from build123d import *

# Parameters (mm, degrees)
EXTRUDE_1_DEPTH     = 20
SKETCH_2_R          = 5
CUT_EXTRUDE_1_DEPTH = 18
CHAMFER_1_SIZE      = 3


with BuildPart() as part:
    # 草圖1 → 填料-伸長1 (new body)
    with BuildSketch(Plane(origin=(0, 0, 0), x_dir=(1, 0, 0), z_dir=(0, 1, 0))):
        Polygon((0, 0), (0, -20), (3.257359313, -23.257359313), (7.5, -19.014718626), (11.742640687, -23.257359313), (15, -20), (15, 0), align=None)
    extrude(amount=EXTRUDE_1_DEPTH)

    # 草圖2 → 除料-伸長1 (cut)
    with BuildSketch(Plane(origin=(0, 0, 0), x_dir=(-1, 0, 0), z_dir=(0, 0, -1))):
        with Locations((-7.5, 10)):
            Circle(SKETCH_2_R)
    extrude(amount=-CUT_EXTRUDE_1_DEPTH, mode=Mode.SUBTRACT)

    # 導角1
    chamfer_1_edges = [part.edges().sort_by_distance(p)[0] for p in [
        (7.5, 20, 0),
        (7.5, 0, 0),
    ]]
    chamfer(chamfer_1_edges, length=CHAMFER_1_SIZE)


solid = part.part
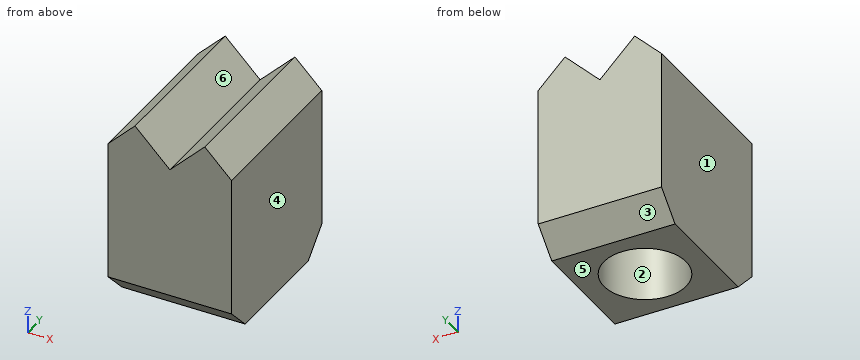
The model under review builds one solid part; all positions refer to its coordinate system, in mm. Face numbers are marked on the shaded views. A direction names the side the tool comes from. Round coordinates to 2 decimals unless told otherwise and drop trailing zeros. Loops run counter-clockwise (first coordinate to the right, second up) from the corner with the lowest first, then second, coordinate; pieces in that order, holes last. Notation, with made-up numbers: M 48.25,24.25 L 87.25,24.25 A26 ccw 87.25,41.25 Z; hole C 82,-16.5 d7. An arc over 180 degrees is marked long. Answer as CSV lines item,"result".
1. For the marked faces 5 and 6, list the 3-axis set-ups (+Z, -Z, +X, -X, +Y, -Y) from which the entire face can be reached by the end or side of a thin tool; tool diameter is ignored.
Outcome:
face 5,"-Z, +X, -X, +Y, -Y"
face 6,"+Z, +Y, -Y"
2. We need section D-D (y = 18.75). Give the boundary of the cut face in (x, z), plus the area to 3 significant figures.
Outcome:
outline,"M 0,1.75 L 15,1.75 L 15,20 L 11.74,23.26 L 7.5,19.01 L 3.26,23.26 L 0,20 Z"
area,"294 mm2"
3. To check wall thickness, follow L1, parallel to Y at x = 7.5, z = 9.5; L2, parallel to Y at x = 4.5, z = 14; L3, parallel to X at y = 8.75, z = 15. State the ranges of each line that lie inside material, in increasing order. Write a range as [from, to].
Outcome:
L1,"y = [0, 5], [15, 20]"
L2,"y = [0, 6], [14, 20]"
L3,"x = [0, 2.66], [12.34, 15]"
4. Insertion check: pin 1 Ø3 at (x, y) = (5.5, 10) entering from -Z. The pin has a flat end and moves straight along its axis. Give the tip position at first contact, or say it passes through.
Outcome:
pin 1,"stops at z = 18"
5. We need section C-C (x = 5.5). Give the boundary of the cut face in (y, z).
Outcome:
outline,"M 0,3 L 3,0 L 5.42,0 L 5.42,18 L 14.58,18 L 14.58,0 L 17,0 L 20,3 L 20,21.01 L 0,21.01 Z"
6. We need section B-B (z = 6.75). Give the boundary of the cut face in (x, y), plus the area to 3 significant figures.
Outcome:
outline,"M 0,0 L 15,0 L 15,20 L 0,20 Z; hole C 7.5,10 d10"
area,"221 mm2"
7. Draft analysis for pull direction X (two halves, no side actions). For the marked faces 1, 2, 3 and 4, state which applies: pulls with the +X half, pulls with the -X half, needs draft (parallel to the pull), parting line crosses it, or undercut.
Outcome:
face 1,"pulls with the -X half"
face 2,"undercut"
face 3,"needs draft"
face 4,"pulls with the +X half"
8. We need section A-A (y = 10). Give the boundary of the cut face in (x, z), plus the area to 3 significant figures.
Outcome:
outline,"M 0,0 L 2.5,0 L 2.5,18 L 12.5,18 L 12.5,0 L 15,0 L 15,20 L 11.74,23.26 L 7.5,19.01 L 3.26,23.26 L 0,20 Z"
area,"140 mm2"
